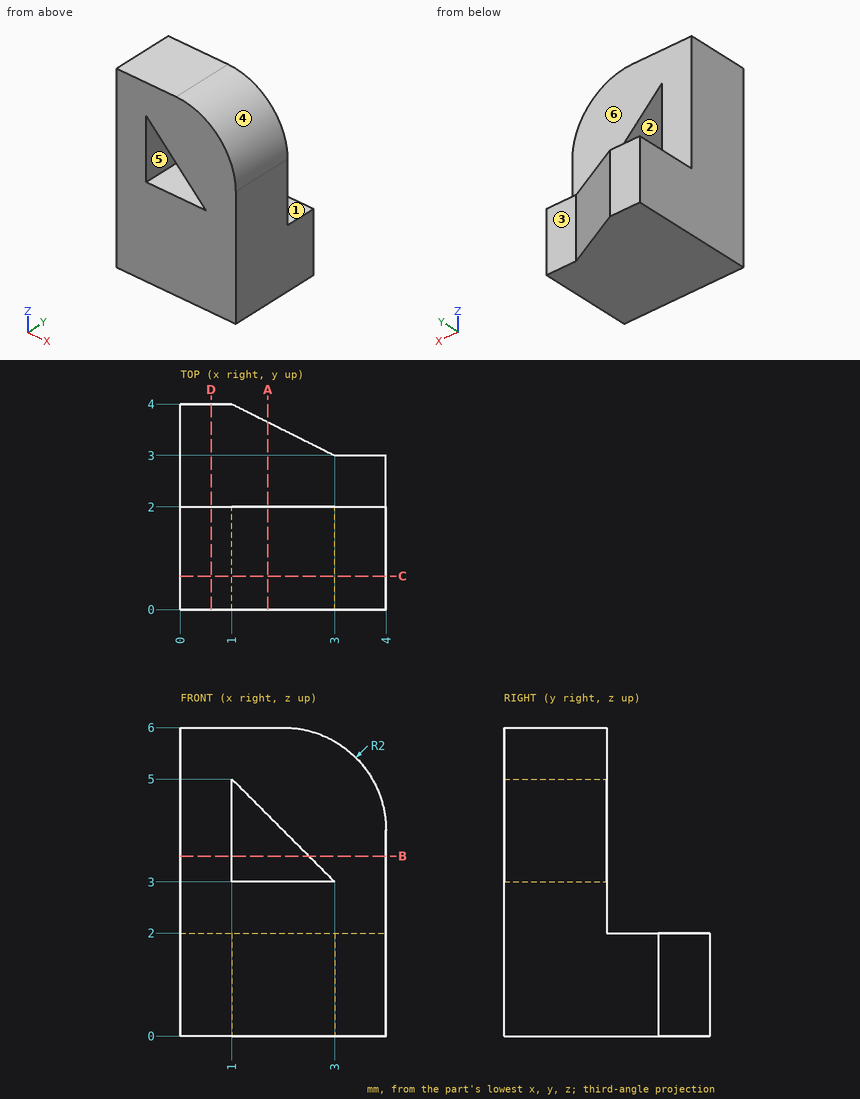
Could you check a few things on this drawing? It's one solid part, dimensions in mm from its lowest x, y, z. A direction names the side the tool comes from. Coordinates: 2 decimals unless noted, no trailing zeros. Write each loop counter-clockwise with the first axis right and the second up, starting at its lowest first coordinate (ties: lowest second). Pieces come first, ordered by that corner, then holes.
Q1. Imagine slicing it at D-D, the plane x = 0.6. List the corners of the cut face in (y, z) for me.
Results found:
outline: (0, 0) - (4, 0) - (4, 2) - (2, 2) - (2, 6) - (0, 6) - close
Q2. Which directions (+Z, -Z, +X, -X, +Y, -Y) give clear straight access to the entire face, cutting with the end or side of a thin tool? Please do the marked faces 1, 2 and 3.
Results found:
face 1: +Z, +X, -X, +Y
face 2: +Y, -Y
face 3: +Z, -Z, +X, +Y
Q3. For P1, Ø1.1, axis at x = 3.5, z = 1.5, coming from the +Y side (3 decimals); P2, Ø0.6, axis at x = 2.5, y = 2.5, coming from the +Z side, each with a flat end and sliding along its axis, tell me the tip position at first contact or that it passes through.
Results found:
P1: stops at y = 3.025
P2: stops at z = 2
Q4. Imagine slicing it at C-C, the plane y = 0.65. List the corners of the cut face in (x, z) for me, plus the area to 3 significant figures.
Results found:
outline: (0, 0) - (4, 0) - (4, 4) arc R2 ccw to (2, 6) - (0, 6) - close; hole (1, 3) - (3, 3) - (1, 5) - close
area: 21.1 mm2
Q5. If we mould it in two halves opening along Z, with no side actions, what happens to the marked faces 4, 5 and 6? For each: +Z half, -Z half, draft (parallel to the pull), parting line (faces both ways), or undercut.
Results found:
face 4: +Z half
face 5: undercut
face 6: draft
Q6. Please list where these lines run through material, in increasing order: L1, parallel to Z at x = 3, y = 2.65; L2, parallel to X at y = 0.4, z = 3.95.
Results found:
L1: z = 0 to 2
L2: x = 0 to 1, 2.05 to 4
Q7. Imagine slicing it at A-A, the plane x = 1.7. List the corners of the cut face in (y, z) for me.
Results found:
outline: (0, 0) - (3.65, 0) - (3.65, 2) - (2, 2) - (2, 3) - (0, 3) - close; (0, 4.3) - (2, 4.3) - (2, 6) - (0, 6) - close
Q8. Imagine slicing it at B-B, the plane z = 3.5. List the corners of the cut face in (x, y) for me.
Results found:
outline: (0, 0) - (1, 0) - (1, 2) - (0, 2) - close; (2.5, 0) - (4, 0) - (4, 2) - (2.5, 2) - close
